For this review, take the finished solid that the model builds, in its own axes (mm). A direction names the side the tool comes from. Coordinates: 2 decimals unless noted, no trailing zeros. Order: outer loops, then holes, each group sorted by start corner. A loop starts at its lowest first (then second) coordinate and runs counter-clockwise, first axis right, second up. Notation, with made-up numbers: (6, 11) -> (57, 11) arc R18 cw to (57, 18) -> close; hole circle Ø3 at (33.5, 53). An arc over 180 degrees is marked (long way). Return JSON: item names as keys, results as strings. Group by question number.
Item 1: For line 1 along X through (y, z) = (2, -30); line 2 along X through (y, z) = (6, -4); line 3 along Z through (x, y) = (-25, 3), list the stretches that pass through material, from the lowest coordinate up.
Item 2: Take a section at A-A (z = -30). Write out the cut boundary in (x, y), then the cut area to 3 significant figures.
Item 3: Machinability: for faces 1 (the flat face through (-48.2, 8.3, -29.8)), 2 (the flat face through (-23.4, 4.8, -6.05)), 3 (the flat face through (-26.36, 3, -3)), 4 (the flat face through (-1, 9, -12.5)), which of the approach directions +Z, -Z, +X, -X, +Y, -Y give a long, thin tool a straight path to every point of the face, cutting with its end or side? Answer none if there is none.
Item 4: Take a section at D-D (x = -14). Write out the cut boundary in (y, z).
Item 5: Draft analysis for pull direction Z (two halves, no side actions). For faces 5 (the cylindrical face through (-24.97, 8.06, -2.98)), 6 (the flat face through (-1.8, 8.3, -29.8)), 7 (the flat face through (-25, 5, -60)), state which applies: +Z half, -Z half, draft (parallel to the pull), parting line (faces both ways), or undercut.
Item 6: Take a section at B-B (x = -25). Write out the cut boundary in (y, z) (3 decimals), then the cut area to 3 significant figures.
Autodesk Inventor part; units mm, degrees
ref_plane "YZ Plane" through (0, 0, 0) normal (1, 0, 0) x (0, 1, 0)
ref_plane "XZ Plane" through (0, 0, 0) normal (0, 1, 0) x (-1, 0, 0)
ref_plane "XY Plane" through (0, 0, 0) normal (0, 0, 1) x (1, 0, 0)
sketch "Sketch1" plane through (0, 0, 0) normal (0, 1, 0) x (-1, 0, 0)
  line L0 (0, 0) -> (50, 0)
  line L1 (50, 0) -> (50, -30)
  line L2 (50, -30) -> (0, -30)
  line L3 (0, -30) -> (0, 0)
  dimension "d0" = 50
  dimension "d1" = 30
extrude "Extrusion1" add sketch "Sketch1" along normal blind 10
sketch "Sketch2" plane through (0, 0, -30) normal (0, 0, -1) x (-1, 0, 0)
  line L0 (50, 10) -> (0, 10)
  line L1 (0, 10) -> (3.5, 10)
  line L2 (3.5, 10) -> (0, 6.5)
  line L3 (0, 0) -> (0, 10)
  line L4 (0, 6.5) -> (0, 10)
extrude "Extrusion2" cut sketch "Sketch2" against normal blind 17.5
sketch "Sketch3" plane through (0, 0, -30) normal (0, 0, -1) x (-1, 0, 0)
  line L0 (50, 0) -> (50, 10)
  line L1 (50, 10) -> (50, 6.5)
  line L2 (50, 6.5) -> (46.5, 10)
  line L3 (50, 10) -> (0, 10)
  line L4 (46.5, 10) -> (50, 10)
  line L5 (50, 10) -> (50, 6.5)
  point P0 (0, 0)
extrude "Extrusion3" cut sketch "Sketch3" against normal blind 17.5
sketch "Sketch4" plane through (0, 0, -30) normal (0, 0, -1) x (-1, 0, 0)
  line L0 (0, 0) -> (50, 0)
  line L1 (3.5, 10) -> (0, 6.5)
  line L2 (0, 0) -> (0, 6.5)
  line L3 (3.5, 10) -> (46.5, 10)
  line L4 (0, 6.5) -> (3.5, 10)
  line L5 (3.5, 10) -> (46.5, 10)
  line L6 (46.5, 10) -> (50, 6.5)
  line L7 (50, 0) -> (50, 10)
  line L8 (50, 6.5) -> (50, 0)
  line L9 (0, 0) -> (0, 10)
  line L10 (50, 0) -> (0, 0)
extrude "Extrusion4" add sketch "Sketch4" along normal blind 30
sketch "Sketch5" plane through (0, 0, -60) normal (0, 0, -1) x (-1, 0, 0)
  line L0 (3.5, 10) -> (0, 6.5)
  line L1 (0, 6.5) -> (3.5, 10)
  line L2 (0, 6.5) -> (0, 10)
  line L3 (3.5, 10) -> (0, 10)
  line L4 (0, 10) -> (0, 6.5)
  point P0 (0, 0)
extrude "Extrusion5" add sketch "Sketch5" against normal blind 12.5
sketch "Sketch6" plane through (0, 0, -60) normal (0, 0, -1) x (-1, 0, 0)
  line L0 (50, 6.5) -> (46.5, 10)
  line L1 (46.5, 10) -> (50, 6.5)
  line L2 (46.5, 10) -> (50, 10)
  line L3 (50, 6.5) -> (50, 10)
  line L4 (50, 10) -> (46.5, 10)
  point P0 (0, 0)
extrude "Extrusion6" add sketch "Sketch6" against normal blind 12.5
fillet "Fillet1" radius 2.5 2 edges at (0, 5, 0) (-50, 5, 0)
sketch "Sketch7" plane through (0, 10, 0) normal (0, 1, 0) x (1, 0, 0)
  line L0 (0, 12.5) -> (0, 47.5)
  circle A0 centre (-25, 30) radius 12.95
  point P0 (0, 0)
  dimension "d21" = 25.9
extrude "Extrusion7" cut sketch "Sketch7" against normal blind 10
sketch "Sketch8" plane through (-47.5, 0, 0) normal (0, 0, 1) x (1, 0, 0)
  line L0 (1, 10) -> (-2.5, 10)
  line L1 (0, 10) -> (45, 10)
  circle A0 centre (22.5, 6.7) radius 1.775
  point P0 (47.5, 0)
  dimension "d26" = 3.55
extrude "Extrusion8" cut sketch "Sketch8" against normal blind 20
sketch "Sketch9" plane through (-47.5, 0, 0) normal (0, 0, 1) x (1, 0, 0)
  circle A0 centre (22.5, 6.7) radius 1.775
  circle A1 centre (22.5, 6.7) radius 1.775
  point P0 (47.5, 0)
extrude "Extrusion9" add sketch "Sketch9" against normal blind 6.05
sketch "Sketch10" plane through (-47.5, 0, 0) normal (0, 0, 1) x (1, 0, 0)
  circle A0 centre (22.5, 6.7) radius 1.775
  circle A1 centre (22.5, 6.7) radius 1.36
  point P0 (47.5, 0)
  dimension "d31" = 2.72
extrude "Extrusion10" cut sketch "Sketch10" against normal blind 6.05 contours A1
sketch "Sketch11" plane through (0, 0, 0) normal (0, -1, 0) x (1, 0, 0)
  line L0 (-23.225, -6.05) -> (-23.225, -17.1722)
  line L1 (-23.225, -17.1722) -> (-26.775, -17.1722)
  line L2 (-26.775, -6.05) -> (-26.775, -17.1722)
  line L3 (-23.225, -6.05) -> (-26.775, -6.05)
  line L4 (-26.775, -6.05) -> (-23.225, -6.05)
  line L5 (-23.225, -6.05) -> (-23.225, -17.1722)
  point P0 (0, 0)
extrude "Extrusion11" cut sketch "Sketch11" against normal blind 6.7
sketch "Sketch12" plane through (0, 0, 0) normal (0, -1, 0) x (1, 0, 0)
  line L0 (-26.36, 0) -> (-26.36, -6.05)
  line L1 (-26.36, 0) -> (-23.64, 0)
  line L2 (-23.64, 0) -> (-23.64, -6.05)
  line L3 (-23.64, -6.05) -> (-26.36, -6.05)
  line L4 (-26.36, 0) -> (-23.64, 0)
  line L5 (-26.36, -6.05) -> (-26.36, 0)
  point P0 (0, 0)
extrude "Extrusion12" cut sketch "Sketch12" against normal blind 6.7
properties part number "SmartWatch_BaseTop"
Findings below:
{
 "1": {"line 1": "x = -50 to -37.95, -12.05 to 0", "line 2": "x = -50 to -26.36, -23.64 to 0", "line 3": "z = -60 to -42.95"},
 "2": {"outline": "(-50, 0) -> (-37.95, 0) -> (-37.95, 10) -> (-46.5, 10) -> (-50, 6.5) -> close; (-12.05, 0) -> (0, 0) -> (0, 6.5) -> (-3.5, 10) -> (-12.05, 10) -> close", "area": "229 mm2"},
 "3": {"face 1": "-X, +Y", "face 2": "-Y", "face 3": "+Z, -Y", "face 4": "+X, +Y"},
 "4": {"outline": "(0, -60) -> (10, -60) -> (10, -36.83) -> (0, -36.83) -> close; (0, -23.17) -> (10, -23.17) -> (10, 0) -> (0, 0) -> close"},
 "5": {"face 5": "draft", "face 6": "undercut", "face 7": "-Z half"},
 "6": {"outline": "(0, -60) -> (10, -60) -> (10, -42.95) -> (0, -42.95) -> close; (8.06, -6.05) -> (8.475, -6.05) -> (8.475, -17.05) -> (10, -17.05) -> (10, 0) -> (8.06, 0) -> close", "area": "199 mm2"}
}
